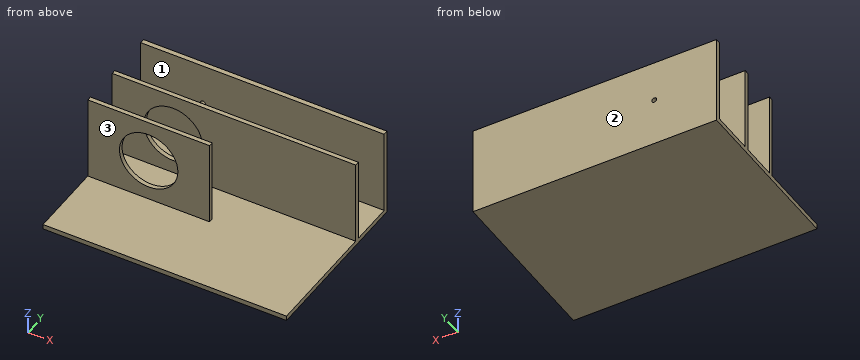
from build123d import *

# Parameters (mm, degrees)
F0_W     = 100
F0_H     = 70
F1_DEPTH = 2
F2_W     = 100
F2_H     = 2
F2_W_2   = 50
F2_H_2   = 1.8
F3_DEPTH = 35
F4_R     = 12
F5_DEPTH = 25
F6_R     = 1
F7_DEPTH = 5.1


with BuildPart() as f1:
    # F0 (on Top) → F1 (new body)
    with BuildSketch(Plane.XY):
        Rectangle(F0_W, F0_H)
    extrude(amount=-F1_DEPTH)

    # F2 (on face) → F3 (join)
    with BuildSketch(Plane.XY):
        with Locations((0, 34)):
            Rectangle(F2_W, F2_H)
        with Locations((-25, 14.1)):
            Rectangle(F2_W_2, F2_H_2)
        with Locations((-25, -2.9)):
            Rectangle(F2_W_2, F2_H_2)
        with Locations((25, 14.1)):
            Rectangle(F2_W_2, F2_H_2)
    extrude(amount=F3_DEPTH)

    # F4 (on face) → F5 (cut)
    with BuildSketch(Plane.XZ.offset(3.8)):
        with Locations((-25, 17.5)):
            Circle(F4_R)
    extrude(amount=-F5_DEPTH, mode=Mode.SUBTRACT)

    # F6 (on face) → F7 (cut)
    with BuildSketch(Plane(origin=(0, 35, 0), x_dir=(-1, 0, 0), z_dir=(0, 1, 0))):
        with Locations((24.412103, 17.940653)):
            Circle(F6_R)
    extrude(amount=-F7_DEPTH, mode=Mode.SUBTRACT)


solid = f1.part
Source: CAD feature listing. Evaluate the final solid. Frame: model axes, mm. Face numbers are marked on the shaded views. A direction names the side the tool comes from. Coordinates: 2 decimals unless noted, no trailing zeros. Order: outer loops, then holes, each group sorted by start corner. A loop starts at its lowest first (then second) coordinate and runs counter-clockwise, first axis right, second up. Notation, with made-up numbers: M 27,7.25 L 42,7.25 A22 cw 42,46.25 Z; hole C 43,81 d10. An arc over 180 degrees is marked long. Write each question's results on one line, items separated by ' | '. Start each with the question number.
Item 1: Set-up query: the marked faces 1, 2 and 3. Return all of +Z, -Z, +X, -X, +Y, -Y with unobstructed straight access to the full face (end or side cutting, diameter ignored); none if empty.
Item 2: Cut plane A-A (z = 3). Return loops of the section in (x, y).
Item 3: First-contact query: pin 1 Ø5.5 at (x, y) = (12, 26) entering from +Z; pin 2 Ø6 at (x, z) = (-38, 28.5) entering from -Y; pin 3 Ø6 at (x, z) = (6, 15.5) entering from -Y; pin 4 Ø6 at (y, z) = (8.5, 3.5) entering from -X. Flat tips, straight axial feed; report the tip coordinate or a pass-through.
Item 4: Cut plane B-B (x = -22). Return loops of the section in (y, z), and give its area (3 significant figures).
Item 5: Cut plane D-D (x = 22). Return loops of the section in (y, z).
Item 6: Cut plane C-C (z = 27). Return loops of the section in (x, y), and give its area (3 significant figures).
Item 7: Line query: probe 1 along Y at (x, z) = (-8, 3); probe 2 along Z at (x, y) = (-25, -2.6); probe 3 along Y at (x, z) = (19, 4). Output: solid intervals per line, ascending.
Checked values:
1) face 1: +Z, +X, -X | face 2: +Z, -Z, +X, -X, +Y | face 3: +Z, +X, -X, -Y
2) outline: M -50,-3.8 L 0,-3.8 L 0,-2 L -50,-2 Z; M -50,13.2 L 50,13.2 L 50,15 L -50,15 Z; M -50,33 L 50,33 L 50,35 L -50,35 Z
3) pin 1: stops at z = 0 | pin 2: stops at y = -3.8 | pin 3: stops at y = 13.2 | pin 4: passes through
4) outline: M -35,-2 L 35,-2 L 35,35 L 33,35 L 33,0 L 15,0 L 15,5.88 L 13.2,5.88 L 13.2,0 L -2,0 L -2,5.88 L -3.8,5.88 L -3.8,0 L -35,0 Z; M -3.8,29.12 L -2,29.12 L -2,35 L -3.8,35 Z; M 13.2,29.12 L 15,29.12 L 15,35 L 13.2,35 Z | area: 252 mm2
5) outline: M -35,-2 L 35,-2 L 35,35 L 33,35 L 33,0 L 15,0 L 15,35 L 13.2,35 L 13.2,0 L -35,0 Z
6) outline: M -50,-3.8 L -32.33,-3.8 L -32.33,-2 L -50,-2 Z; M -50,13.2 L -32.33,13.2 L -32.33,15 L -50,15 Z; M -50,33 L 50,33 L 50,35 L -50,35 Z; M -17.67,-3.8 L 0,-3.8 L 0,-2 L -17.67,-2 Z; M -17.67,13.2 L 50,13.2 L 50,15 L -17.67,15 Z | area: 417 mm2
7) probe 1: y = -3.8 to -2, 13.2 to 15, 33 to 35 | probe 2: z = -2 to 5.5, 29.5 to 35 | probe 3: y = 13.2 to 15, 33 to 35
